```python
from build123d import *

# Parameters (mm, degrees)
SKETCH1_R           = 30.25
SKETCH1_R_2         = 25.25
EXTRUDE_THIN1_DEPTH = 1
SKETCH2_R           = 1.65
CUT_EXTRUDE3_DEPTH  = 10
BOSS_EXTRUDE1_DEPTH = 1


with BuildPart() as part:
    # Sketch1 → Extrude-Thin1 (new body)
    with BuildSketch(Plane(origin=(0, 0, 0), x_dir=(1, 0, 0), z_dir=(0, 1, 0))):
        Circle(SKETCH1_R)
        Circle(SKETCH1_R_2, mode=Mode.SUBTRACT)
    extrude(amount=-EXTRUDE_THIN1_DEPTH)

    # Sketch2 → Cut-Extrude3 (cut)
    with BuildSketch(Plane(origin=(0, 0, 0), x_dir=(1, 0, 0), z_dir=(0, 1, 0))):
        with Locations((0, 27.5)):
            Circle(SKETCH2_R)
        with Locations((23.815698604, -13.75)):
            Circle(SKETCH2_R)
        with Locations((-23.815698604, -13.75)):
            Circle(SKETCH2_R)
    extrude(amount=-CUT_EXTRUDE3_DEPTH, mode=Mode.SUBTRACT)

    # Sketch5 → Boss-Extrude1 (add)
    with BuildSketch(Plane.XZ.offset(1)):
        with BuildLine():
            Line((0, 56.75), (0, 30.25))
            ThreePointArc((0, 30.25), (1.319486468, 30.221208703), (2.636461218, 30.134889617))
            Line((2.636461218, 30.134889617), (4.946088401, 56.534049117))
            ThreePointArc((4.946088401, 56.534049117), (2.475400233, 56.695986575), (0, 56.75))
        make_face()
        with BuildLine():
            Line((15.310966763, 54.645556057), (8.161352328, 29.128247942))
            ThreePointArc((8.161352328, 29.128247942), (9.424140859, 28.744531116), (10.668990002, 28.306097441))
            Line((10.668990002, 28.306097441), (20.015377938, 53.103174538))
            ThreePointArc((20.015377938, 53.103174538), (17.679999793, 53.925690606), (15.310966763, 54.645556057))
        make_face()
        with BuildLine():
            Line((29.486389165, 48.488301208), (15.717414489, 25.846186988))
            ThreePointArc((15.717414489, 25.846186988), (16.829849835, 25.136003154), (17.910248605, 24.377971509))
            Line((17.910248605, 24.377971509), (33.600218458, 45.733880434))
            ThreePointArc((33.600218458, 45.733880434), (31.573354649, 47.155972858), (29.486389165, 48.488301208))
        make_face()
        with BuildLine():
            Line((41.474940973, 38.734890878), (22.107787919, 20.647232582))
            ThreePointArc((22.107787919, 20.647232582), (22.98736584, 19.663252827), (23.823186003, 18.641842952))
            Line((23.823186003, 18.641842952), (44.693084485, 34.972713638))
            ThreePointArc((44.693084485, 34.972713638), (43.125058229, 36.888912328), (41.474940973, 38.734890878))
        make_face()
        with BuildLine():
            Line((50.387486144, 26.108690891), (26.858527857, 13.916967391))
            ThreePointArc((26.858527857, 13.916967391), (27.440014081, 12.732168992), (27.969266679, 11.523134184))
            Line((27.969266679, 11.523134184), (52.471268894, 21.61778066))
            ThreePointArc((52.471268894, 21.61778066), (51.478373524, 23.885969926), (50.387486144, 26.108690891))
        make_face()
        with BuildLine():
            Line((55.563021976, 11.546128741), (29.617293652, 6.154544395))
            ThreePointArc((29.617293652, 6.154544395), (29.857562008, 4.856798428), (30.040994796, 3.549807269))
            Line((30.040994796, 3.549807269), (56.357899329, 6.659555785))
            ThreePointArc((56.357899329, 6.659555785), (56.013773353, 9.111514406), (55.563021976, 11.546128741))
        make_face()
        with BuildLine():
            Line((56.617702652, -3.872756958), (30.179480268, -2.064333004))
            ThreePointArc((30.179480268, -2.064333004), (30.060711149, -3.378778657), (29.884719758, -4.686792612))
            Line((29.884719758, -4.686792612), (56.06472219, -8.792577876))
            ThreePointArc((56.06472219, -8.792577876), (56.394887858, -6.338700456), (56.617702652, -3.872756958))
        make_face()
        with BuildLine():
            Line((53.47330733, -19.004417991), (28.503392894, -10.130108268))
            ThreePointArc((28.503392894, -10.130108268), (28.034394863, -11.363767186), (27.512031768, -12.575794526))
            Line((27.512031768, -12.575794526), (51.613481086, -23.59260626))
            ThreePointArc((51.613481086, -23.59260626), (52.59345152, -21.318802902), (53.47330733, -19.004417991))
        make_face()
        with BuildLine():
            Line((46.363041428, -32.72660828), (24.713339264, -17.444579744))
            ThreePointArc((24.713339264, -17.444579744), (23.928895759, -18.505957088), (23.098902242, -19.532107291))
            Line((23.098902242, -19.532107291), (43.334304206, -36.642878967))
            ThreePointArc((43.334304206, -36.642878967), (44.891399482, -34.717787264), (46.363041428, -32.72660828))
        make_face()
        with BuildLine():
            Line((35.814240841, -44.021615747), (19.090410316, -23.465266544))
            ThreePointArc((19.090410316, -23.465266544), (18.048699924, -24.275644812), (16.972632807, -25.039813011))
            Line((16.972632807, -25.039813011), (31.841220224, -46.97551697))
            ThreePointArc((31.841220224, -46.97551697), (33.859957709, -45.541912168), (35.814240841, -44.021615747))
        make_face()
        with BuildLine():
            Line((22.609261849, -52.05174136), (12.051632968, -27.745641871))
            ThreePointArc((12.051632968, -27.745641871), (10.829914583, -28.244919014), (9.587580841, -28.690430349))
            Line((9.587580841, -28.690430349), (17.986618602, -53.824195779))
            ThreePointArc((17.986618602, -53.824195779), (20.317277772, -52.988401787), (22.609261849, -52.05174136))
        make_face()
        with BuildLine():
            Line((7.727457336, -56.221427438), (4.119041135, -29.968249868))
            ThreePointArc((4.119041135, -29.968249868), (2.807924021, -30.119396785), (1.491461864, -30.213209719))
            Line((1.491461864, -30.213209719), (2.798031761, -56.680980216))
            ThreePointArc((2.798031761, -56.680980216), (5.267758287, -56.504984051), (7.727457336, -56.221427438))
        make_face()
        with BuildLine():
            Line((-7.727457336, -56.221427438), (-4.119041135, -29.968249868))
            ThreePointArc((-4.119041135, -29.968249868), (-5.42231742, -29.760056683), (-6.715272016, -29.49521354))
            Line((-6.715272016, -29.49521354), (-12.598072295, -55.333995649))
            ThreePointArc((-12.598072295, -55.333995649), (-10.172446731, -55.830850141), (-7.727457336, -56.221427438))
        make_face()
        with BuildLine():
            Line((-22.609261849, -52.05174136), (-12.051632968, -27.745641871))
            ThreePointArc((-12.051632968, -27.745641871), (-13.250410384, -27.193549321), (-14.423964891, -26.589692304))
            Line((-14.423964891, -26.589692304), (-27.059834961, -49.88314176))
            ThreePointArc((-27.059834961, -49.88314176), (-24.858207911, -51.015997486), (-22.609261849, -52.05174136))
        make_face()
        with BuildLine():
            Line((-35.814240841, -44.021615747), (-19.090410316, -23.465266544))
            ThreePointArc((-19.090410316, -23.465266544), (-20.095781026, -22.610220807), (-21.062898275, -21.71213523))
            Line((-21.062898275, -21.71213523), (-39.514693459, -40.732683448))
            ThreePointArc((-39.514693459, -40.732683448), (-37.700349529, -42.417521679), (-35.814240841, -44.021615747))
        make_face()
        with BuildLine():
            Line((-46.363041428, -32.72660828), (-24.713339264, -17.444579744))
            ThreePointArc((-24.713339264, -17.444579744), (-25.450739522, -16.349995651), (-26.139692851, -15.224288412))
            Line((-26.139692851, -15.224288412), (-49.038927911, -28.561268343))
            ThreePointArc((-49.038927911, -28.561268343), (-47.74642869, -30.673132337), (-46.363041428, -32.72660828))
        make_face()
        with BuildLine():
            Line((-53.47330733, -19.004417991), (-28.503392894, -10.130108268))
            ThreePointArc((-28.503392894, -10.130108268), (-28.918133096, -8.877166114), (-29.277825989, -7.607325769))
            Line((-29.277825989, -7.607325769), (-54.926169417, -14.271594625))
            ThreePointArc((-54.926169417, -14.271594625), (-54.25137366, -16.65385709), (-53.47330733, -19.004417991))
        make_face()
        with BuildLine():
            Line((-56.617702652, -3.872756958), (-30.179480268, -2.064333004))
            ThreePointArc((-30.179480268, -2.064333004), (-30.240801031, -0.745957776), (-30.24455671, 0.573837425))
            Line((-30.24455671, 0.573837425), (-56.739788209, 1.076537978))
            ThreePointArc((-56.739788209, 1.076537978), (-56.73274243, -1.399441448), (-56.617702652, -3.872756958))
        make_face()
        with BuildLine():
            Line((-55.563021976, 11.546128741), (-29.617293652, 6.154544395))
            ThreePointArc((-29.617293652, 6.154544395), (-29.320647095, 7.440574837), (-28.96818702, 8.712441722))
            Line((-28.96818702, 8.712441722), (-54.345276476, 16.344828685))
            ThreePointArc((-54.345276476, 16.344828685), (-55.006503229, 13.958764363), (-55.563021976, 11.546128741))
        make_face()
        with BuildLine():
            Line((-50.387486144, 26.108690891), (-26.858527857, 13.916967391))
            ThreePointArc((-26.858527857, 13.916967391), (-26.225914898, 15.075274053), (-25.54337942, 16.204884073))
            Line((-25.54337942, 16.204884073), (-47.9202242, 30.40089822))
            ThreePointArc((-47.9202242, 30.40089822), (-49.200683321, 28.281712479), (-50.387486144, 26.108690891))
        make_face()
        with BuildLine():
            Line((-41.474940973, 38.734890878), (-22.107787919, 20.647232582))
            ThreePointArc((-22.107787919, 20.647232582), (-21.186126568, 21.591909157), (-20.22413622, 22.495484305))
            Line((-20.22413622, 22.495484305), (-37.941148116, 42.202272209))
            ThreePointArc((-37.941148116, 42.202272209), (-39.745873809, 40.507135361), (-41.474940973, 38.734890878))
        make_face()
        with BuildLine():
            Line((-29.486389165, 48.488301208), (-15.717414489, 25.846186988))
            ThreePointArc((-15.717414489, 25.846186988), (-14.575060151, 26.507171136), (-13.404961357, 27.117697377))
            Line((-13.404961357, 27.117697377), (-25.148150645, 50.873696731))
            ThreePointArc((-25.148150645, 50.873696731), (-27.343294663, 49.72832932), (-29.486389165, 48.488301208))
        make_face()
        with BuildLine():
            Line((-15.310966763, 54.645556057), (-8.161352327, 29.128247942))
            ThreePointArc((-8.161352327, 29.128247942), (-6.883028198, 29.456517493), (-5.591601834, 29.728714889))
            Line((-5.591601834, 29.728714889), (-10.490029886, 55.772051899))
            ThreePointArc((-10.490029886, 55.772051899), (-12.912788438, 55.261400586), (-15.310966763, 54.645556057))
        make_face()
    extrude(amount=-BOSS_EXTRUDE1_DEPTH)


solid = part.part
```
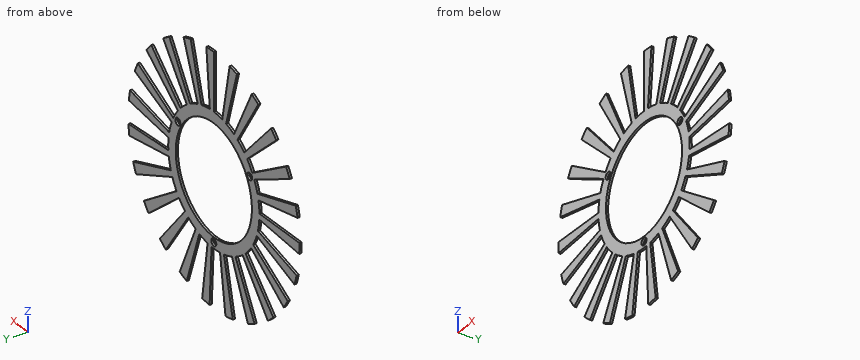
Source: CAD feature listing. Evaluate the final solid. Frame: model axes, mm. Round coordinates to 2 decimals unless told otherwise and drop trailing zeros. Write each loop counter-clockwise with the first axis right and the second up, starting at its lowest first coordinate (ties: lowest second). Pieces come first, ordered by that corner, then holes. Notation, with made-up numbers: M 10,-11.5 L 14,-11.5 A20 cw 14,22.5 Z; hole C 19,55.25 d7. An arc over 180 degrees is marked long. Use CSV: the item, a comma, the result in double quotes. Start each with the question number.
Q1. Line query: line 1 (X direction, y = -0.5, z = 0); line 2 (X direction, y = -0.7, z = -41); line 3 (X direction, y = -0.75, z = -44.5). Output: solid intervals per line, ascending. Write a range as from..to.
Q2. Cut plane B-B on x = 39. Output: boundary loops of the cut face in (y, z), plus the area to 3 significant figures.
Q3. Cut plane A-A on x = -43. Output: boundary loops of the cut face in (y, z).
Q4. Cut plane C-C on y = -0.8. Count the separate pieces of the cut face and the enclosed holes in it, plus the area to 3 significant figures.
Results found:
1,line 1,"-56.75..-25.25, 25.25..30.25"
1,line 2,"-39.24..-33.36, -22.24..-17.81, -9.33..-5.64, 2.02..5.64, 13.7..17.81, 27.79..33.36"
1,line 3,"-24.14..-19.33, -10.13..-6.12, 2.2..6.12, 14.87..19.33, 30.16..35.22"
2,outline,"M -1,-32.98 L 0,-32.98 L 0,-27.53 L -1,-27.53 Z; M -1,-17.83 L 0,-17.83 L 0,-13.86 L -1,-13.86 Z; M -1,-6.12 L 0,-6.12 L 0,-2.67 L -1,-2.67 Z; M -1,4.61 L 0,4.61 L 0,8.1 L -1,8.1 Z; M -1,16.07 L 0,16.07 L 0,20.21 L -1,20.21 Z; M -1,30.52 L 0,30.52 L 0,36.42 L -1,36.42 Z"
2,area,"26.4 mm^2"
3,outline,"M -1,-30.35 L 0,-30.35 L 0,-25.04 L -1,-25.04 Z; M -1,-15.28 L 0,-15.28 L 0,-11.17 L -1,-11.17 Z; M -1,-2.94 L 0,-2.94 L 0,0.82 L -1,0.82 Z; M -1,8.94 L 0,8.94 L 0,12.93 L -1,12.93 Z; M -1,22.28 L 0,22.28 L 0,27.28 L -1,27.28 Z"
4,separate pieces,"1"
4,enclosed holes,"4"
4,area,"3,160 mm^2"
